```python
from build123d import *

# Parameters (mm, degrees)
SKETCH1_R           = 30
SKETCH1_R_2         = 15
BOSS_EXTRUDE3_DEPTH = 40
BOSS_EXTRUDE4_DEPTH = 30
BOSS_EXTRUDE5_DEPTH = 20
BOSS_EXTRUDE6_DEPTH = 6
SKETCH11_R          = 10
CUT_EXTRUDE1_DEPTH  = 60


with BuildPart() as part:
    # Sketch1 → Boss-Extrude3 (new body, symmetric)
    with BuildSketch(Plane.XY):
        Circle(SKETCH1_R)
        Circle(SKETCH1_R_2, mode=Mode.SUBTRACT)
    extrude(amount=BOSS_EXTRUDE3_DEPTH, both=True)

    # Sketch4 → Boss-Extrude4 (add, symmetric)
    with BuildSketch(Plane.XY):
        with BuildLine():
            Line((0, 30), (0, 66))
            Line((0, 66), (40, 66))
            Line((40, 66), (40, 46))
            Line((40, 46), (20, 46))
            Line((20, 46), (20, 22.360679775))
            ThreePointArc((20, 22.360679775), (10.704662693, 28.025170769), (0, 30))
        make_face()
    extrude(amount=BOSS_EXTRUDE4_DEPTH, both=True)

    # Sketch5 → Boss-Extrude5 (add)
    with BuildSketch(Plane(origin=(0, 66, 0), x_dir=(1, 0, 0), z_dir=(0, 1, 0))):
        with BuildLine():
            Line((40, 30), (40, -30))
            ThreePointArc((40, -30), (70, 0), (40, 30))
        make_face()
    extrude(amount=-BOSS_EXTRUDE5_DEPTH)

    # Sketch9 → Boss-Extrude6 (add, symmetric)
    with BuildSketch(Plane.XY):
        with BuildLine():
            Line((0, 66), (-26.721706285, 13.636363636))
            ThreePointArc((-26.721706285, 13.636363636), (-15.666989036, 25.584085963), (0, 30))
            Line((0, 30), (0, 66))
        make_face()
    extrude(amount=BOSS_EXTRUDE6_DEPTH, both=True)

    # Sketch10 → Revolve1 (revolve)
    with BuildSketch(Plane.XY, mode=Mode.PRIVATE) as revolve1_sk:
        Polygon((20, 66), (45, 66), (45, 106), (25, 106), align=None)
    revolve(revolve1_sk.sketch.rotate(Axis((45, 66, 0), (0, 1, 0)), 270), axis=Axis((45, 66, 0), (0, 1, 0)))  # turned: the seam where the file's is

    # Sketch11 → Cut-Extrude1 (cut)
    with BuildSketch(Plane(origin=(0, 106, 0), x_dir=(1, 0, 0), z_dir=(0, 1, 0))):
        with Locations(Location((45, 0, 0), (0, 0, 270))):  # turned: the seam where the file's is
            Circle(SKETCH11_R)
    extrude(amount=-CUT_EXTRUDE1_DEPTH, mode=Mode.SUBTRACT)


solid = part.part
```
Verification items for the finished model (mm, model axes). A direction names the side the tool comes from. Coordinates: 2 decimals unless noted, no trailing zeros. Loops run counter-clockwise (first coordinate to the right, second up) from the corner with the lowest first, then second, coordinate; pieces in that order, holes last. Notation, with made-up numbers: (-11, -29.75) - (30, -29.75) arc R20 cw to (30, -24.75) - close; hole circle Ø7 at (50, -5.5). An arc over 180 degrees is marked (long way). Put each result on its own line as item: value.
Item 1: Section check B-B (x = -12.5). Enter the section's corners in (y, z), then the cut area to 3 significant figures.
Conclusion:
outline: (-27.27, -40) - (-8.29, -40) - (-8.29, 40) - (-27.27, 40) - close; (8.29, -40) - (27.27, -40) - (27.27, -6) - (41.51, -6) - (41.51, 6) - (27.27, 6) - (27.27, 40) - (8.29, 40) - close
area: 3,210 mm2
Item 2: Set-up check for faces 1 (the face through (-14.985, 0.66, -0.56)), 2 (the face through (6, 14, -40)), 3 (the face through (-6.503, -29.287, 0.56)), 4 (the face through (-7, 40, 6)), 5 (the face through (-7, 40, -6)): record each of +Z, -Z, +X, -X, +Y, -Y from which the full face is reachable in a straight line by a thin tool's end or side.
Conclusion:
face 1: +Z, -Z
face 2: -Z, +X, -X, +Y, -Y
face 3: none
face 4: +Z, -X, +Y
face 5: -Z, -X, +Y
Item 3: Section check D-D (x = 45). Enter the section's corners in (y, z).
Conclusion:
outline: (46, -29.58) - (66, -29.58) - (66, -25) - (106, -20) - (106, -10) - (46, -10) - close; (46, 10) - (106, 10) - (106, 20) - (66, 25) - (66, 29.58) - (46, 29.58) - close
Item 4: Section check C-C (y = 62). Enter the section's corners in (x, z).
Conclusion:
outline: (-2.04, -6) - (0, -6) - (0, -30) - (40, -30) arc R30 ccw to (40, 30) - (0, 30) - (0, 6) - (-2.04, 6) - close; hole circle Ø20 at (45, 0)
Item 5: Draft check along Y on faces 6 (the face through (20, 34, 0)), 7 (the face through (35.24, 76.42, -2.17)), 8 (the face through (23.208, 90.164, 2.861)), 9 (the face through (34, 46, 0)). Enter one of: pulls with the +Y half, pulls with the -Y half, needs draft (parallel to the pull), parting line crosses it, or undercut.
Conclusion:
face 6: undercut
face 7: needs draft
face 8: pulls with the +Y half
face 9: undercut
Item 6: Section check A-A (y = 0). Enter the section's corners in (x, z).
Conclusion:
outline: (-30, -40) - (-15, -40) - (-15, 40) - (-30, 40) - close; (15, -40) - (30, -40) - (30, 40) - (15, 40) - close
Item 7: Gauge pin test, flat ends, axial feed: pin 1 Ø1.5 at (x, z) = (35, 3.5) entering from -Y; pin 2 Ø4 at (x, z) = (3.5, -3.5) entering from -Y; pin 3 Ø5 at (x, z) = (10, -11.5) entering from -Y. Record the tip position at first contact, or that the pin passes through.
Conclusion:
pin 1: stops at y = 46
pin 2: stops at y = -29.96
pin 3: stops at y = -29.05
Item 8: Scan lines: line 1 along Y through (x, z) = (0, 5); line 2 along X through (y, z) = (0.5, -11.5); line 3 along X through (y, z) = (66.5, 0). Record each from-to range of solid material in increasing order.
Conclusion:
line 1: y = -30 to -15, 15 to 66
line 2: x = -30 to -14.99, 14.99 to 30
line 3: x = 20.06 to 35, 55 to 69.94
